Autodesk Inventor part; units mm, degrees
ref_plane "YZ Plane" through (0, 0, 0) normal (1, 0, 0) x (0, 1, 0)
ref_plane "XZ Plane" through (0, 0, 0) normal (0, 1, 0) x (-1, 0, 0)
ref_plane "XY Plane" through (0, 0, 0) normal (0, 0, 1) x (1, 0, 0)
sketch "Sketch1" plane through (0, 0, 0) normal (0, 0, 1) x (1, 0, 0)
  line L0 (-13.5, 9) -> (13.5, 9)
  line L1 (13.5, 9) -> (13.5, -9)
  line L2 (13.5, -9) -> (-13.5, -9)
  line L3 (-13.5, -9) -> (-13.5, 9)
  line L4 (-13.5, 9) -> (13.5, -9) construction
  line L5 (13.5, 9) -> (-13.5, -9) construction
  point P0 (0, 0)
  dimension "c14_inside_outer_width" = 27
  dimension "c14_inside_outer_height" = 18
extrude "Extrusion1" add sketch "Sketch1" along normal blind 20
chamfer "Chamfer1" distance 4 angle 45 2 edges at (-13.5, 9, 10) (13.5, 9, 10)
sketch "Sketch2" plane through (0, 0, 20) normal (0, 0, 1) x (1, 0, 0)
  line L0 (-2, 8.5) -> (2, 8.5)
  line L1 (3, 7.5) -> (3, -2.5)
  line L2 (2, -3.5) -> (-2, -3.5)
  line L3 (-3, -2.5) -> (-3, 7.5)
  line L4 (-3, 8.5) -> (3, -3.5) construction
  line L5 (3, 8.5) -> (-3, -3.5) construction
  line L6 (9.5, 9) -> (-9.5, 9) construction
  line L7 (0, 9) -> (0, -9)
  line L8 (-13.5, -9) -> (13.5, -9) construction
  arc A0 (-2, 8.5) -> (-3, 7.5) centre (-2, 7.5) ccw
  arc A1 (3, 7.5) -> (2, 8.5) centre (2, 7.5) ccw
  arc A2 (2, -3.5) -> (3, -2.5) centre (2, -2.5) ccw
  arc A3 (-3, -2.5) -> (-2, -3.5) centre (-2, -2.5) ccw
  line L9 (-10, 3.5) -> (-6, 3.5)
  line L10 (-5, 2.5) -> (-5, -7.5)
  line L11 (-6, -8.5) -> (-10, -8.5)
  line L12 (-11, -7.5) -> (-11, 2.5)
  line L13 (-11, 3.5) -> (-5, -8.5) construction
  line L14 (-5, 3.5) -> (-11, -8.5) construction
  arc A4 (-10, 3.5) -> (-11, 2.5) centre (-10, 2.5) ccw
  arc A5 (-5, 2.5) -> (-6, 3.5) centre (-6, 2.5) ccw
  arc A6 (-6, -8.5) -> (-5, -7.5) centre (-6, -7.5) ccw
  arc A7 (-11, -7.5) -> (-10, -8.5) centre (-10, -7.5) ccw
  line L15 (6, -8.5) -> (10, -8.5)
  arc A8 (10, -8.5) -> (11, -7.5) centre (10, -7.5) ccw
  line L16 (5, 2.5) -> (5, -7.5)
  line L17 (11, -7.5) -> (11, 2.5)
  line L18 (11, 3.5) -> (5, -8.5) construction
  line L19 (5, 3.5) -> (11, -8.5) construction
  arc A9 (6, 3.5) -> (5, 2.5) centre (6, 2.5) ccw
  line L20 (10, 3.5) -> (6, 3.5)
  arc A10 (11, 2.5) -> (10, 3.5) centre (10, 2.5) ccw
  arc A11 (5, -7.5) -> (6, -8.5) centre (6, -7.5) ccw
  point P0 (0, 0)
  point P1 (0, 2.5)
  point P2 (-8, -2.5)
  point P3 (8, -2.5)
  dimension "d7" = 6
  dimension "d8" = 12
  dimension "d9" = 0.5
  dimension "d10" = 1
  dimension "d11" = 6
  dimension "d12" = 12
  dimension "d13" = 1
  dimension "d14" = 0.5
  dimension "d15" = 2
extrude "Extrusion2" add sketch "Sketch2" along normal blind 1
sketch "Sketch3" plane through (0, 0, 0) normal (0, 0, -1) x (-1, 0, 0)
  line L0 (-13.5, 5) -> (-9.5, 9) construction
  line L1 (-13.5, -9) -> (-13.5, 5) construction
  line L2 (13.5, -9) -> (-13.5, -9) construction
  line L3 (13.5, 5) -> (13.5, -9) construction
  line L4 (9.5, 9) -> (13.5, 5) construction
  line L5 (-9.5, 9) -> (9.5, 9) construction
  line L6 (0, 9) -> (0, -9)
  line L7 (-15.25, 11) -> (15.25, 11)
  line L8 (15.25, 11) -> (15.25, -11)
  line L9 (15.25, -11) -> (-15.25, -11)
  line L10 (-15.25, -11) -> (-15.25, 11)
  line L11 (-15.25, 11) -> (15.25, -11) construction
  line L12 (15.25, 11) -> (-15.25, -11) construction
  line L13 (-13.5, -9) -> (-13.5, 9) construction
  line L14 (-13.5, 0) -> (13.5, 0) construction
  point P0 (0, 0)
  point P1 (0, 0)
  dimension "c14_outer_width_1" = 30.5
  dimension "c14_outer_height" = 22
extrude "Extrusion3" add sketch "Sketch3" along normal blind 4
fillet "Fillet1" radius 3 4 edges at (-15.25, 11, -2) (-15.25, -11, -2) (15.25, -11, -2) (15.25, 11, -2)
sketch "Sketch5" plane through (0, 0, 0) normal (0, 0, 1) x (1, 0, 0)
  line L0 (-12.25, 11) -> (12.25, 11)
  arc A0 (-12.25, 11) -> (-15.25, 8) centre (-12.25, 8) ccw construction
  line L1 (-15.25, -8) -> (-15.25, 8) construction
  arc A1 (-15.25, -8) -> (-12.25, -11) centre (-12.25, -8) ccw construction
  line L2 (12.25, -11) -> (-12.25, -11)
  arc A2 (12.25, -11) -> (15.25, -8) centre (12.25, -8) ccw construction
  line L3 (15.25, 8) -> (15.25, -8) construction
  arc A3 (15.25, 8) -> (12.25, 11) centre (12.25, 8) ccw construction
  line L4 (0, 11) -> (0, -11)
  arc A4 (-12.25, 11) -> (-13.8922, 10.5106) centre (-12.25, 8) ccw
  line L5 (-13.8922, 10.5106) -> (-22.2844, 5.0212)
  line L6 (-15.25, 0) -> (15.25, 0)
  arc A5 (-22.2844, 5.0212) -> (-25, 0) centre (-19, 0) ccw
  line L7 (-15.25, 0) -> (-70.2247, 0)
  arc A6 (-13.8922, -10.5106) -> (-12.25, -11) centre (-12.25, -8) ccw
  line L8 (-13.8922, -10.5106) -> (-22.2844, -5.0212)
  arc A7 (-25, 0) -> (-22.2844, -5.0212) centre (-19, 0) ccw
  arc A8 (13.8922, 10.5106) -> (12.25, 11) centre (12.25, 8) ccw
  line L9 (13.8922, 10.5106) -> (22.2844, 5.0212)
  arc A9 (25, 0) -> (22.2844, 5.0212) centre (19, 0) ccw
  arc A10 (12.25, -11) -> (13.8922, -10.5106) centre (12.25, -8) ccw
  line L10 (13.8922, -10.5106) -> (22.2844, -5.0212)
  arc A11 (22.2844, -5.0212) -> (25, 0) centre (19, 0) ccw
  point P0 (0, 0)
  dimension "d26" = 50
  dimension "d27" = 3
  dimension "d28" = 6
extrude "Extrusion5" add sketch "Sketch5" against normal blind 2
sketch "Sketch6" plane through (0, 0, -2) normal (0, 0, -1) x (-1, 0, 0)
  arc A0 (22.2844, -5.0212) -> (22.2844, 5.0212) centre (19, 0) ccw construction
  arc A1 (-22.2844, 5.0212) -> (-22.2844, -5.0212) centre (-19, 0) ccw construction
  line L0 (-25, 0) -> (25, 0) construction
  line L1 (0, 10) -> (0, -11) construction
  line L2 (-12.25, -11) -> (12.25, -11) construction
  point P0 (0, 0)
  point P1 (-20.5, 0)
  point P2 (20.5, 0)
  dimension "d55" = 41
hole "Hole1" at (20.5, 0, -2) at (-20.5, 0, -2) direction (0, 0, 1) diameter 4 end through all countersink diameter 6 countersink angle 90
fillet "Fillet3" radius 3 6 edges at (-13.5, 5, 10) (-9.5, 9, 10) (-13.5, -9, 10) (13.5, -9, 10) (13.5, 5, 10) (9.5, 9, 10)
sketch "Sketch7" plane through (0, 0, -4) normal (0, 0, -1) x (-1, 0, 0)
  line L0 (10.5, -9) -> (-10.5, -9) construction
  arc A0 (-13.5, -6) -> (-10.5, -9) centre (-10.5, -6) ccw construction
  line L1 (-13.5, -6) -> (-13.5, 3.7574) construction
  arc A1 (-12.6213, 5.8787) -> (-13.5, 3.7574) centre (-10.5, 3.7574) ccw construction
  line L2 (-10.3787, 8.1213) -> (-12.6213, 5.8787) construction
  arc A2 (-8.2574, 9) -> (-10.3787, 8.1213) centre (-8.2574, 6) ccw construction
  line L3 (-8.2574, 9) -> (8.2574, 9) construction
  arc A3 (10.3787, 8.1213) -> (8.2574, 9) centre (8.2574, 6) ccw construction
  line L4 (12.6213, 5.8787) -> (10.3787, 8.1213) construction
  arc A4 (13.5, 3.7574) -> (12.6213, 5.8787) centre (10.5, 3.7574) ccw construction
  line L5 (13.5, 3.7574) -> (13.5, -6) construction
  arc A5 (10.5, -9) -> (13.5, -6) centre (10.5, -6) ccw construction
  arc A6 (-11.9142, 5.1716) -> (-12.5, 3.7574) centre (-10.5, 3.7574) ccw
  line L6 (-12.5, 3.7574) -> (-12.5, -6)
  arc A7 (-12.5, -6) -> (-10.5, -8) centre (-10.5, -6) ccw
  line L7 (-10.5, -8) -> (10.5, -8)
  arc A8 (10.5, -8) -> (12.5, -6) centre (10.5, -6) ccw
  line L8 (12.5, -6) -> (12.5, 3.7574)
  arc A9 (12.5, 3.7574) -> (11.9142, 5.1716) centre (10.5, 3.7574) ccw
  line L9 (11.9142, 5.1716) -> (9.6716, 7.4142)
  arc A10 (9.6716, 7.4142) -> (8.2574, 8) centre (8.2574, 6) ccw
  line L10 (8.2574, 8) -> (-8.2574, 8)
  arc A11 (-8.2574, 8) -> (-9.6716, 7.4142) centre (-8.2574, 6) ccw
  line L11 (-9.6716, 7.4142) -> (-11.9142, 5.1716)
  point P0 (0, 0)
  dimension "d40" = 1
extrude "Extrusion6" cut sketch "Sketch7" against normal blind 21
fillet "Fillet4" radius 0.5 12 edges at (0, 8, -4) (-9.0227, 7.8478, -4) (-10.7929, 6.2929, -4) (-12.3478, 4.5227, -4) (-12.5, -1.1213, -4) (-11.9142, -7.4142, -4) (0, -8, -4) (11.9142, -7.4142, -4) (12.5, -1.1213, -4) (12.3478, 4.5227, -4) (10.7929, 6.2929, -4) (9.0227, 7.8478, -4)
sketch "Sketch8" plane through (0, 0, 21) normal (0, 0, 1) x (1, 0, 0)
  line L0 (-6, 3.5) -> (-10, 3.5) construction
  arc A0 (-10, 3.5) -> (-11, 2.5) centre (-10, 2.5) ccw construction
  line L1 (-11, 2.5) -> (-11, -7.5) construction
  arc A1 (-11, -7.5) -> (-10, -8.5) centre (-10, -7.5) ccw construction
  line L2 (-10, -8.5) -> (-6, -8.5) construction
  arc A2 (-6, -8.5) -> (-5, -7.5) centre (-6, -7.5) ccw construction
  line L3 (-5, -7.5) -> (-5, 2.5) construction
  arc A3 (-5, 2.5) -> (-6, 3.5) centre (-6, 2.5) ccw construction
  line L4 (-8, 3.5) -> (-8, -8.5)
  line L5 (-11, -2.5) -> (-5, -2.5)
  line L6 (-8.25, -0.1) -> (-7.75, -0.1)
  line L7 (-7.75, -0.1) -> (-7.75, -4.9)
  line L8 (-7.75, -4.9) -> (-8.25, -4.9)
  line L9 (-8.25, -4.9) -> (-8.25, -0.1)
  line L10 (-8.25, -0.1) -> (-7.75, -4.9) construction
  line L11 (-7.75, -0.1) -> (-8.25, -4.9) construction
  point P0 (0, 0)
  point P1 (-8, -2.5)
  dimension "d44" = 0.5
  dimension "d45" = 4.8
extrude "Extrusion7" add sketch "Sketch8" along normal blind 10
chamfer "Chamfer2" distance 1.2 angle 45 2 edges at (-8, -0.1, 31) (-8, -4.9, 31)
sketch "Sketch9" plane through (-7.75, -4.9, 21) normal (1, 0, 0) x (0, 0, -1)
  line L0 (-10, 1.2) -> (-10, 3.6) construction
  line L1 (-10, 2.4) -> (0.0273, 2.4)
  circle A0 centre (-7, 2.4) radius 2.05
  point P0 (21, 4.9)
  dimension "d51" = 4.1
  dimension "d52" = 3
extrude "Extrusion8" cut sketch "Sketch9" against normal blind 10
equation "\"d27\" = c14_outer_fillet"
equation "\"d39\" = c14_outer_fillet"
properties part number "my_C14"
Build history of the part. All positions in model axes, mm. A direction names the side the tool comes from. Round coordinates to 2 decimals unless told otherwise and drop trailing zeros. Loops run counter-clockwise (first coordinate to the right, second up) from the corner with the lowest first, then second, coordinate; pieces in that order, holes last. Notation, with made-up numbers: (39.5, 6.25) -> (49.5, 6.25) arc R13 cw to (49.5, 27.25) -> close; hole circle Ø9 at (37.25, 44.5). An arc over 180 degrees is marked (long way). Answer in a Markdown table with one row per item.
Item 1: Saw through at C-C (x = -20.5). Write the cut outline in (y, z).
Answers below:
| item | result |
|---|---|
| outline | (-6.19, -2) -> (-3, -2) -> (-2, -1) -> (-2, 0) -> (-6.19, 0) -> close; (2, -1) -> (3, -2) -> (6.19, -2) -> (6.19, 0) -> (2, 0) -> close |
Item 2: Pin check, flat tips, straight feed: pin 1 (1.1 mm diameter, centred on y = -2, z = 20.5, fed in from -X); pin 2 (1.6 mm diameter, centred on y = -0.5, z = -3, fed in from -X); pin 3 (8.5 mm diameter, centred on x = 0, z = 13.5, fed in from +Y). Stop position of each tip, or through.
Answers below:
| item | result |
|---|---|
| pin 1 | stops at x = -13.5 |
| pin 2 | stops at x = -15.25 |
| pin 3 | stops at y = 9 |
Item 3: Saw through at A-A (z = 8). Write the cut outline in (x, y), and give its area (3 significant figures).
Answers below:
| item | result |
|---|---|
| outline | (-13.5, -6) arc R3 ccw to (-10.5, -9) -> (10.5, -9) arc R3 ccw to (13.5, -6) -> (13.5, 3.76) arc R3 ccw to (12.62, 5.88) -> (10.38, 8.12) arc R3 ccw to (8.26, 9) -> (-8.26, 9) arc R3 ccw to (-10.38, 8.12) -> (-12.62, 5.88) arc R3 ccw to (-13.5, 3.76) -> close; hole (-12.5, -6) arc R2 ccw to (-10.5, -8) -> (10.5, -8) arc R2 ccw to (12.5, -6) -> (12.5, 3.76) arc R2 ccw to (11.91, 5.17) -> (9.67, 7.41) arc R2 ccw to (8.26, 8) -> (-8.26, 8) arc R2 ccw to (-9.67, 7.41) -> (-11.91, 5.17) arc R2 ccw to (-12.5, 3.76) -> close |
| area | 79.1 mm² |
Item 4: Mould opens along Y. For faces 1 (the cylindrical face through (-2.715, 8.199, 20.493)), 2 (the flat face through (5, -2.4, 20.5)), 3 (the cylindrical face through (12.344, 4.533, 6.607)) say: +Y half, -Y half, draft (parallel to the pull), parting line (faces both ways), or undercut.
Answers below:
| item | result |
|---|---|
| face 1 | +Y half |
| face 2 | draft |
| face 3 | undercut |
Item 5: Drill centre lines: L1, parallel to X at y = 0, z = -0.55; L2, parallel to X at y = -0.75, z = 2.5; L3, parallel to Y at x = -8, z = 28. Where is each one in solid material? Low to high. Write a range as [from, to].
Answers below:
| item | result |
|---|---|
| L1 | x = [-25, -22.5], [-18.5, -12.5], [12.5, 18.5], [22.5, 25] |
| L2 | x = [-13.5, -12.5], [12.5, 13.5] |
| L3 | y = [-4.9, -4.55], [-0.45, -0.1] |
Item 6: Which spindle directions (+Z, -Z, +X, -X, +Y, -Y) get a long thin tool onto all of the face, cutting with end or side? Do faces 4 (the flat face through (11, -2.6, 20.5)), 5 (the flat face through (-8, 3.5, 20.5)), 6 (the cylindrical face through (9.421, 8.765, 10.14)), 7 (the flat face through (-8.25, -3, 25)), 8 (the cylindrical face through (-10.88, 6.41, -3.85)). Say none if no direction does.
Answers below:
| item | result |
|---|---|
| face 4 | +Z, +X, +Y, -Y |
| face 5 | +Z, -X, +Y |
| face 6 | +Z, +X, +Y |
| face 7 | +Z, -X, +Y, -Y |
| face 8 | -Z |
Item 7: Saw through at B-B (z = 26.5). Write the cut outline in (x, y), and give its area (3 significant figures).
Answers below:
| item | result |
|---|---|
| outline | (-8.25, -4.9) -> (-7.75, -4.9) -> (-7.75, -3.9) -> (-8.25, -3.9) -> close; (-8.25, -1.1) -> (-7.75, -1.1) -> (-7.75, -0.1) -> (-8.25, -0.1) -> close |
| area | 1.00 mm² |
